from build123d import *

# Parameters (mm, degrees)
F0_R     = 2
F1_DEPTH = 6


with BuildPart() as f1:
    # F0 (on Right) → F1 (new body)
    with BuildSketch(Plane.YZ):
        with BuildLine():
            Line((-158.73, 250), (-150, 250))
            Line((-150, 250), (-150, 260))
            Line((-150, 260), (-135, 260))
            Line((-135, 260), (-135, 270))
            Line((-135, 270), (-180, 270))
            Line((-180, 270), (-180, 105))
            Line((-180, 105), (-170, 105))
            Line((-170, 105), (-170, 120))
            Line((-170, 120), (-160, 120))
            Line((-160, 120), (-160, 248.73))
            ThreePointArc((-160, 248.73), (-159.628026, 249.628026), (-158.73, 250))
        make_face()
        with Locations((-170, 140)):
            Circle(F0_R, mode=Mode.SUBTRACT)
        with Locations((-170, 260)):
            Circle(F0_R, mode=Mode.SUBTRACT)
    extrude(amount=F1_DEPTH)


solid = f1.part
Geometry check sheet. Reference: the model listing, model coordinates, mm. A direction names the side the tool comes from. Round coordinates to 2 decimals unless told otherwise and drop trailing zeros. Order: outer loops, then holes, each group sorted by start corner. A loop starts at its lowest first (then second) coordinate and runs counter-clockwise, first axis right, second up. Notation, with made-up numbers: M -23,35 L 22,35 A28 ccw 22,69 Z; hole C 32,-21.75 d6. An arc over 180 degrees is marked long. Answer in a Markdown table with one row per item.
(1) Draft check along Y on faces 3 (the face through (3, -135, 265)), 4 (the face through (3, -171.6, 138.8)), 5 (the face through (0, -168, 207)). Enter one of: released by +Y, released by -Y, zero draft, split by the parting line, or undercut.
Responses:
| item | result |
|---|---|
| face 3 | released by +Y |
| face 4 | undercut |
| face 5 | zero draft |
(2) Sectioned sample at C-C, the plane y = -139.5. Record the cut outline in (x, z).
Responses:
| item | result |
|---|---|
| outline | M 0,260 L 6,260 L 6,270 L 0,270 Z |
(3) Tool access check on faces 1 (the face through (3, -160, 183)), 2 (the face through (3, -171.6, 258.8)). Record the directions out of +Z, -Z, +X, -X, +Y, -Y that give a thin tool (end or side, any length) a straight path to the whole face; none if there is none.
Responses:
| item | result |
|---|---|
| face 1 | -Z, +X, -X, +Y |
| face 2 | +X, -X |
(4) Sectioned sample at A-A, the plane z = 140. Record the cut outline in (x, y), and give its area (3 significant figures).
Responses:
| item | result |
|---|---|
| outline | M 0,-180 L 6,-180 L 6,-172 L 0,-172 Z; M 0,-168 L 6,-168 L 6,-160 L 0,-160 Z |
| area | 96.0 mm² |
(5) Scan lines: probe 1 along Y at (x, z) = (3.65, 251); probe 2 along Y at (x, z) = (1.85, 136); probe 3 along Z at (x, y) = (3.8, -167.5). Record each from-to range of solid material in increasing order. Write a range as from..to.
Responses:
| item | result |
|---|---|
| probe 1 | y = -180..-150 |
| probe 2 | y = -180..-160 |
| probe 3 | z = 120..270 |
(6) Sectioned sample at D-D, the plane z = 256. Record the cut outline in (x, y), and give its area (3 significant figures).
Responses:
| item | result |
|---|---|
| outline | M 0,-180 L 6,-180 L 6,-150 L 0,-150 Z |
| area | 180 mm² |
(7) Go/stop test with flat-tipped pins: P1, Ø1.8, axis at x = 3, y = -145, coming from the -Z side; P2, Ø3, axis at x = 3.5, y = -166, coming from the -Z side; P3, Ø1.8, axis at x = 2.5, y = -155.5, coming from the -Z side. Record where each tip stops, or that it passes through.
Responses:
| item | result |
|---|---|
| P1 | stops at z = 260 |
| P2 | stops at z = 120 |
| P3 | stops at z = 250 |
(8) Sectioned sample at B-B, the plane x = 1.15. Record the cut outline in (y, z), and give its area (3 significant figures).
Responses:
| item | result |
|---|---|
| outline | M -180,105 L -170,105 L -170,120 L -160,120 L -160,248.73 A1.27 cw -158.73,250 L -150,250 L -150,260 L -135,260 L -135,270 L -180,270 Z; hole C -170,140 d4; hole C -170,260 d4 |
| area | 3,480 mm² |
